from build123d import *

# Parameters (mm, degrees)
SKETCH1_W           = 82.042
SKETCH1_H           = 56.388
SKETCH1_R           = 1.651
BOSS_EXTRUDE1_DEPTH = 2.54
SKETCH2_W           = 19.05
SKETCH2_H           = 2.7432
SKETCH2_W_2         = 2.7432
SKETCH2_H_2         = 19.05
BOSS_EXTRUDE2_DEPTH = 2.54


with BuildPart() as part:
    # Sketch1 → Boss-Extrude1 (new body)
    with BuildSketch(Plane(origin=(0, 0, 0), x_dir=(1, 0, 0), z_dir=(0, 1, 0))):
        Rectangle(SKETCH1_W, SKETCH1_H)
        with Locations((-34.671, 21.844)):
            Circle(SKETCH1_R, mode=Mode.SUBTRACT)
        with Locations((-34.671, -21.844)):
            Circle(SKETCH1_R, mode=Mode.SUBTRACT)
        with Locations((34.671, -21.844)):
            Circle(SKETCH1_R, mode=Mode.SUBTRACT)
        with Locations((34.671, 21.844)):
            Circle(SKETCH1_R, mode=Mode.SUBTRACT)
    extrude(amount=BOSS_EXTRUDE1_DEPTH)

    # Sketch2 → Boss-Extrude2 (add)
    with BuildSketch(Plane(origin=(0, 2.54, 0), x_dir=(1, 0, 0), z_dir=(0, 1, 0))):
        with Locations((0, 29.5656)):
            Rectangle(SKETCH2_W, SKETCH2_H)
        with Locations((0, -29.5656)):
            Rectangle(SKETCH2_W, SKETCH2_H)
        with Locations((42.3926, 0)):
            Rectangle(SKETCH2_W_2, SKETCH2_H_2)
        with Locations((-42.3926, 0)):
            Rectangle(SKETCH2_W_2, SKETCH2_H_2)
    extrude(amount=-BOSS_EXTRUDE2_DEPTH)


solid = part.part
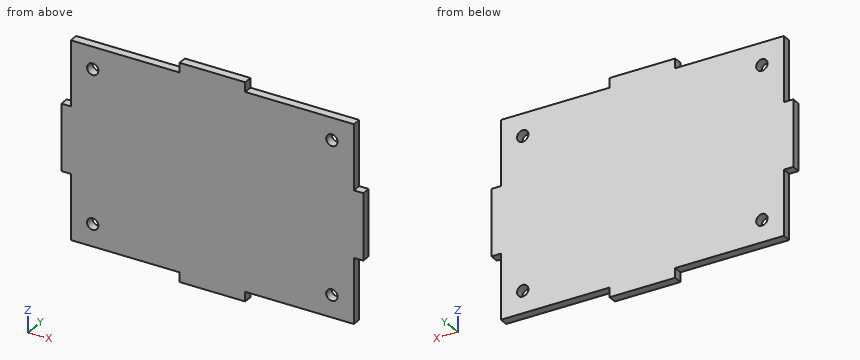
Can you work these out from the model? Positions are in its coordinate system, mm. Round coordinates to 2 decimals unless told otherwise and drop trailing zeros. Loops run counter-clockwise (first coordinate to the right, second up) from the corner with the lowest first, then second, coordinate; pieces in that order, holes last. Notation, with made-up numbers: (73, -33.75) - (119, -33.75) arc R37 cw to (119, 3.25) - close; hole circle Ø8 at (-22.75, 12.25). An arc over 180 degrees is marked (long way). Answer in a Markdown table with one row per item. Add a question column.
Q1. For pin 1 Ø0.8 at (x, y) = (-42, 1) entering from -Z (3 decimals); pin 2 Ø1.3 at (y, z) = (1, -19.5) entering from +X; pin 3 Ø1.3 at (x, y) = (-22.5, 1.5) entering from +Z; pin 4 Ø2 at (x, z) = (-34.671, -21.844) entering from -Y, each with a flat end and sliding along its axis, tell me the tip position at first contact or that it passes through.
Q2. I want a section at B-B on x = -26.5. List the corners of the cut face in (y, z) for me.
Q3. I want a section at A-A on y = 0.7. List the corners of the cut face in (x, z) for me (3 decimals).
Q4. I want a section at C-C on z = -14. List the corners of the cut face in (x, y) for me.
Q5. I need wall thicknesses on L1, parallel to X at y = 1.5, z = -11.5; L2, parallel to Z at x = -37, y = 0.6; L3, parallel to X at y = 1.55, z = -21.5. Which ranges of each line are inside material? Lowest first, please.
A:
| question | item | result |
|---|---|---|
| 1 | pin 1 | z = -9.525 |
| 1 | pin 2 | x = 41.02 |
| 1 | pin 3 | z = 28.19 |
| 1 | pin 4 | through |
| 2 | outline | (0, -28.19) - (2.54, -28.19) - (2.54, 28.19) - (0, 28.19) - close |
| 3 | outline | (-43.764, -9.525) - (-41.021, -9.525) - (-41.021, -28.194) - (-9.525, -28.194) - (-9.525, -30.937) - (9.525, -30.937) - (9.525, -28.194) - (41.021, -28.194) - (41.021, -9.525) - (43.764, -9.525) - (43.764, 9.525) - (41.021, 9.525) - (41.021, 28.194) - (9.525, 28.194) - (9.525, 30.937) - (-9.525, 30.937) - (-9.525, 28.194) - (-41.021, 28.194) - (-41.021, 9.525) - (-43.764, 9.525) - close; hole circle Ø3.302 at (-34.671, -21.844); hole circle Ø3.302 at (-34.671, 21.844); hole circle Ø3.302 at (34.671, -21.844); hole circle Ø3.302 at (34.671, 21.844) |
| 4 | outline | (-41.02, 0) - (41.02, 0) - (41.02, 2.54) - (-41.02, 2.54) - close |
| 5 | L1 | -41.02 to 41.02 |
| 5 | L2 | -28.19 to 28.19 |
| 5 | L3 | -41.02 to -36.29, -33.06 to 33.06, 36.29 to 41.02 |
